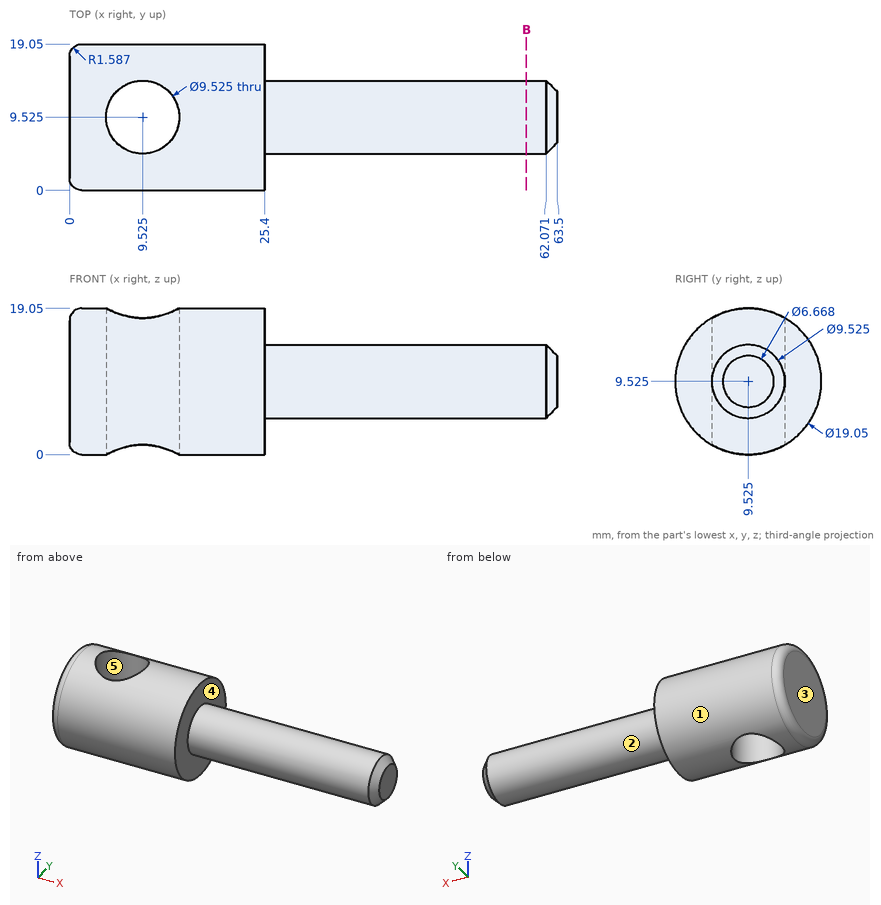
Source: three-view drawing plus pictorial views. Frame: mm from the lowest corner of the part. A direction names the side the tool comes from. Round coordinates to 2 decimals unless told otherwise and drop trailing zeros. Order: outer loops, then holes, each group sorted by start corner. A loop starts at its lowest first (then second) coordinate and runs counter-clockwise, first axis right, second up. Notation, with made-up numbers: M -17,59 L 2,59 A14 cw 2,77 Z; hole C 43.25,67 d7. An arc over 180 degrees is marked long. One line per item, written item: value.
(1) Pull-direction query (X, two-part tool) for the marked faces 3, 4 and 5; classes: pulls with the +X half, pulls with the -X half, needs draft (parallel to the pull), parting line crosses it, or undercut.
Result sheet:
face 3: pulls with the -X half
face 4: pulls with the +X half
face 5: undercut
(2) Pin query (flat end, axial travel): P1, Ø3, axis at x = 25.5, z = 11.5, coming from the -Y side; P2, Ø3, axis at x = 26, y = 14.5, coming from the -Z side; P3, Ø1, axis at x = 25, z = 4.5, coming from the -Y side. Return the tip coordinate at first contact, or that it passes through.
Result sheet:
P1: y = 0.01
P2: z = 0.71
P3: y = 1.14
(3) Line query: probe 1 along Z at (x, y) = (61, 9.5); probe 2 along X at (y, z) = (12, 1.5) (1 decimal); probe 3 along X at (y, z) = (16, 14). Output: solid intervals per line, ascending. Write a range as [from, to].
Result sheet:
probe 1: [4.76, 14.29]
probe 2: [0.1, 5.5], [13.6, 25.4]
probe 3: [0, 25.4]
(4) Cut plane B-B (x = 59.5). Return the cut outline in (y, z) (1 decimal).
Result sheet:
outline: C 9.5,9.5 d9.5
(5) Reachability of the marked faces 1 and 2 from +Z, -Z, +X, -X, +Y, -Y: full face, straight path, thin tool, end or side. Return the list, or none.
Result sheet:
face 1: +X, -X
face 2: +X
